from build123d import *

# Parameters (mm, degrees)
BOSS_EXTRUDE1_DEPTH = 12
CUT_EXTRUDE1_DEPTH  = 3.5
SKETCH3_W           = 1.4
SKETCH3_H           = 12
BOSS_EXTRUDE2_DEPTH = 7
SKETCH4_R           = 1.25
CUT_EXTRUDE2_DEPTH  = 3.5
SKETCH5_W           = 7
SKETCH5_H           = 1.4
BOSS_EXTRUDE3_DEPTH = 12
CUT_EXTRUDE3_DEPTH  = 3.5
CUT_EXTRUDE4_DEPTH  = 3.5


with BuildPart() as part:
    # Sketch1 → Boss-Extrude1 (new body)
    with BuildSketch(Plane.XY):
        Polygon((0, 0), (0, 7), (4.5, 7), (11, 4.5), (11, 0), align=None)
    extrude(amount=BOSS_EXTRUDE1_DEPTH)

    # Sketch2 → Cut-Extrude1 (cut)
    with BuildSketch(Plane.ZY):
        Polygon((4.443375673, 1.4), (4.443375673, 6.4), (1.556624327, 6.4), (0.113248654, 3.9), (3, 3.9), (3, 1.4), align=None)
        Polygon((4.443375673, 6.4), (4.443375673, 1.4), (5.886751346, 3.9), align=None)
        Polygon((10.443375673, 6.4), (7.556624327, 6.4), (7.556624327, 1.4), (9, 1.4), (9, 3.9), (11.886751346, 3.9), align=None)
        Polygon((9, 3.9), (9, 1.4), (10.443375673, 1.4), (11.886751346, 3.9), align=None)
        Polygon((1.556624327, 1.4), (3, 1.4), (3, 3.9), (0.113248654, 3.9), align=None)
        Polygon((7.556624327, 6.4), (7.556624327, 1.4), (6.113248654, 3.9), align=None)
        Polygon((0.113248654, 3.9), (1.556624327, 6.4), (0, 6.4), (0, 3.9), align=None)
        Polygon((1.556624327, 1.4), (0.113248654, 3.9), (0, 3.9), (0, 1.4), align=None)
        Polygon((12, 6.4), (10.443375673, 6.4), (11.886751346, 3.9), (12, 3.9), align=None)
        Polygon((12, 3.9), (11.886751346, 3.9), (10.443375673, 1.4), (12, 1.4), align=None)
    extrude(amount=-CUT_EXTRUDE1_DEPTH, mode=Mode.SUBTRACT)

    # Sketch3 → Boss-Extrude2 (add)
    with BuildSketch(Plane(origin=(0, 7, 0), x_dir=(1, 0, 0), z_dir=(0, 1, 0))):
        with Locations((0.7, -6)):
            Rectangle(SKETCH3_W, SKETCH3_H)
    extrude(amount=-BOSS_EXTRUDE2_DEPTH)

    # Sketch4 → Cut-Extrude2 (cut)
    # profile 1 of 2: a face of its own
    with BuildSketch(Plane.XZ):
        Polygon((7.5, 6.113248654), (10, 7.556624327), (10, 12), (5, 12), (5, 7.556624327), align=None)
    # profile 2 of 2: a face of its own
    with BuildSketch(Plane.XZ):
        Polygon((5, 4.443375673), (5, 0), (10, 0), (10, 4.443375673), (7.5, 5.886751346), align=None)
        with Locations(Location((7.5, 3, 0), (0, 0, 270))):
            Circle(SKETCH4_R, mode=Mode.SUBTRACT)
    extrude(amount=-CUT_EXTRUDE2_DEPTH, mode=Mode.SUBTRACT)

    # Sketch5 → Boss-Extrude3 (add)
    with BuildSketch(Plane(origin=(0, 0, 0), x_dir=(-1, 0, 0), z_dir=(0, 0, -1))):
        with Locations((-7.5, 0.7)):
            Rectangle(SKETCH5_W, SKETCH5_H)
    extrude(amount=-BOSS_EXTRUDE3_DEPTH)

    # Sketch6 → Cut-Extrude3 (cut)
    with BuildSketch(Plane.ZY):
        with BuildLine():
            ThreePointArc((2.25, 3.9), (2.616116524, 3.016116524), (3.5, 2.65))
            Line((3.5, 2.65), (3.5, 3.9))
            Line((3.5, 3.9), (2.25, 3.9))
        make_face()
        with BuildLine():
            Line((3.5, 3.9), (3.5, 2.65))
            ThreePointArc((3.5, 2.65), (4.383883476, 3.016116524), (4.75, 3.9))
            ThreePointArc((4.75, 3.9), (3.5, 5.15), (2.25, 3.9))
            Line((2.25, 3.9), (3.5, 3.9))
        make_face()
        with BuildLine():
            ThreePointArc((9.75, 3.9), (7.616116524, 4.783883476), (8.5, 2.65))
            Line((8.5, 2.65), (8.5, 3.9))
            Line((8.5, 3.9), (9.75, 3.9))
        make_face()
        with BuildLine():
            Line((8.5, 3.9), (8.5, 2.65))
            ThreePointArc((8.5, 2.65), (9.383883476, 3.016116524), (9.75, 3.9))
            Line((9.75, 3.9), (8.5, 3.9))
        make_face()
    extrude(amount=-CUT_EXTRUDE3_DEPTH, mode=Mode.SUBTRACT)

    # Sketch4_3 → Cut-Extrude4 (cut)
    with BuildSketch(Plane.XZ):
        with BuildLine():
            ThreePointArc((7.5, 10.25), (6.616116524, 8.116116524), (8.75, 9))
            Line((8.75, 9), (7.5, 9))
            Line((7.5, 9), (7.5, 10.25))
        make_face()
        with BuildLine():
            Line((7.5, 9), (8.75, 9))
            ThreePointArc((8.75, 9), (8.383883476, 9.883883476), (7.5, 10.25))
            Line((7.5, 10.25), (7.5, 9))
        make_face()
        with BuildLine():
            ThreePointArc((7.5, 1.75), (8.383883476, 2.116116524), (8.75, 3))
            Line((8.75, 3), (7.5, 3))
            Line((7.5, 3), (7.5, 1.75))
        make_face()
        with BuildLine():
            Line((7.5, 3), (8.75, 3))
            ThreePointArc((8.75, 3), (6.616116524, 3.883883476), (7.5, 1.75))
            Line((7.5, 1.75), (7.5, 3))
        make_face()
    extrude(amount=-CUT_EXTRUDE4_DEPTH, mode=Mode.SUBTRACT)


solid = part.part
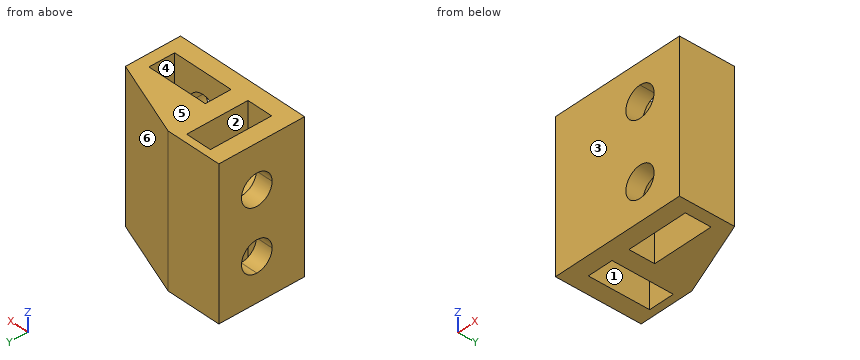
CAD build for the part. Positions are in the model's coordinates, mm. Face numbers are marked on the shaded views. A direction names the side the tool comes from. Give positions to 0.01 mm unless a question says otherwise; leave off trailing zeros. Write each loop counter-clockwise with the first axis right and the second up, starting at its lowest first coordinate (ties: lowest second). Pieces come first, ordered by that corner, then holes. Notation, with made-up numbers: (-11.75, 23.5) - (17.25, 23.5) arc R19 cw to (17.25, 32.5) - close; hole circle Ø3 at (39, -35). An arc over 180 degrees is marked (long way). Put each result on its own line as item: value.
(1) Tool access for the marked faces 1, 2 and 3: list every direction of +Z, -Z, +X, -X, +Y, -Y with a clear straight run to the whole face (end or side of a thin tool).
Working result:
face 1: -Z
face 2: +Z
face 3: +Z, -Z, +X, -X, -Y
(2) Wall check: L1, parallel to Z at x = 7.5, y = 1.1; L2, parallel to X at y = 2.5, z = 3.75; L3, parallel to Z at x = 0.7, y = 3.9. Give the ranges that are in metal, low to high.
Working result:
L1: 0 to 1.75, 4.25 to 7.75, 10.25 to 12
L2: 0 to 1.4, 3.5 to 5, 10 to 11
L3: 0 to 2.25, 4.75 to 7.25, 9.75 to 12
(3) Drop flat-ended pins along their axis: pin 1 Ø1.5 at (x, z) = (7.5, 3) entering from -Y; pin 2 Ø4 at (x, z) = (9.5, 2) entering from +Y; pin 3 Ø1.5 at (x, z) = (6.5, 4.5) entering from +Y. Give the stop position or say it passes through.
Working result:
pin 1: y = 3.5
pin 2: y = 5.85
pin 3: y = 6.52
(4) Saw through at C-C (z = 8.25). List the corners of the cut face in (x, y), then the cut area to 3 significant figures.
Working result:
outline: (0, 0) - (6.5, 0) - (6.5, 1.4) - (5, 1.4) - (5, 3.5) - (10, 3.5) - (10, 1.4) - (8.5, 1.4) - (8.5, 0) - (11, 0) - (11, 4.5) - (4.5, 7) - (0, 7) - (0, 5.12) - (1.4, 5.12) - (1.4, 6.4) - (3.5, 6.4) - (3.5, 1.4) - (1.4, 1.4) - (1.4, 2.68) - (0, 2.68) - close
area: 41.6 mm^2
(5) Saw through at A-A (y = 5). List the corners of the cut face in (x, z), then the cut area to 3 significant figures.
Working result:
outline: (0, 0) - (1.4, 0) - (1.4, 2.91) - (0, 2.91) - close; (0, 4.09) - (1.4, 4.09) - (1.4, 5.25) - (3.5, 5.25) - (3.5, 0) - (9.7, 0) - (9.7, 12) - (3.5, 12) - (3.5, 6.75) - (1.4, 6.75) - (1.4, 7.91) - (0, 7.91) - close; (0, 9.09) - (1.4, 9.09) - (1.4, 12) - (0, 12) - close
area: 91.0 mm^2
(6) Pull direction X, two halves, no side cores. Call the marked faces 4, 5 and 6: released by +X, released by -X, zero draft, split by the parting line, or undercut.
Working result:
face 4: undercut
face 5: zero draft
face 6: released by +X
(7) Saw through at B-B (x = 2.25). List the corners of the cut face in (y, z), then the cut area to 3 significant figures.
Working result:
outline: (0, 0) - (1.4, 0) - (1.4, 4.44) - (3.9, 5.89) - (6.4, 4.44) - (6.4, 0) - (7, 0) - (7, 12) - (6.4, 12) - (6.4, 7.56) - (3.9, 6.11) - (1.4, 7.56) - (1.4, 12) - (0, 12) - close
area: 32.3 mm^2
(8) Saw through at D-D (z = 5.25). List the corners of the cut face in (x, y), then the cut area to 3 significant figures.
Working result:
outline: (0, 0) - (11, 0) - (11, 4.5) - (4.5, 7) - (0, 7) - close; hole (1.4, 2.8) - (3.5, 2.8) - (3.5, 5) - (1.4, 5) - close; hole (6.4, 1.4) - (8.6, 1.4) - (8.6, 3.5) - (6.4, 3.5) - close
area: 59.6 mm^2
